Source: CAD feature listing. Evaluate the final solid. Frame: model axes, mm. Face numbers are marked on the shaded views. A direction names the side the tool comes from. Give positions to 0.01 mm unless a question says otherwise; leave off trailing zeros. Write each loop counter-clockwise with the first axis right and the second up, starting at its lowest first coordinate (ties: lowest second). Pieces come first, ordered by that corner, then holes.
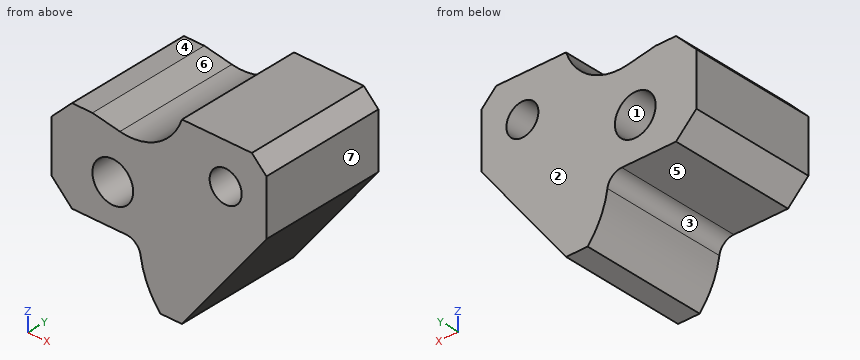
```python
from build123d import *

# Parameters (mm, degrees)
F0_R     = 7
F1_DEPTH = 43
F2_R     = 5.5
F3_DEPTH = 43.001


with BuildPart() as f1:
    # F0 (on Front) → F1 (new body)
    with BuildSketch(Plane.XZ):
        with BuildLine():
            Line((-14, 18), (-21, 11))
            Line((-21, 11), (-21, -7))
            Line((-21, -7), (-14, -14))
            Line((-14, -14), (4.616354, -14))
            ThreePointArc((4.616354, -14), (7.88159, -15.213414), (9.561993, -18.264706))
            ThreePointArc((9.561993, -18.264706), (11.898823, -26.115672), (16.337795, -33))
            Line((16.337795, -33), (23.746698, -33))
            Line((23.746698, -33), (52.746698, 5))
            Line((52.746698, 5), (52.746698, 24))
            Line((52.746698, 24), (47.746698, 29))
            Line((47.746698, 29), (23.746698, 29))
            ThreePointArc((23.746698, 29), (15.440895, 18.713813), (2.43554, 16.33626))
            Line((2.43554, 16.33626), (-7, 18))
            Line((-7, 18), (-14, 18))
        make_face()
        Circle(F0_R, mode=Mode.SUBTRACT)
    extrude(amount=F1_DEPTH)

    # F2 (on face) → F3 (cut, through all)
    with BuildSketch(Plane.XZ.offset(43)):
        with Locations((38.746698, 15)):
            Circle(F2_R)
    extrude(amount=-F3_DEPTH, mode=Mode.SUBTRACT)


solid = f1.part
```
1. Line query: L1, parallel to Z at x = 0, y = -9; L2, parallel to X at y = -34.5, z = 14; L3, parallel to X at y = -15, z = -3. Output: solid intervals per line, ascending.
2. Mould query, pull axis Z, two halves, no side actions, for the marked faces 1, 2 and 3. Classes: +Z half, -Z half, draft (parallel to the pull), parting line (faces both ways), or undercut.
3. Contact query for flat-ended pins moving along their axis: P1, Ø8, axis at y = -33.5, z = -21.5, coming from the -X side; P2, Ø6, axis at x = 44.5, z = 5.5, coming from the +Y side; P3, Ø1.5, axis at x = -4.5, y = -16, coming from the +Z side; P4, Ø10, axis at y = -10, z = -9, coming from the +X side. Output: stop coordinate, or through.
4. Cut plane C-C, the plane x = 0. Return the cut outline in (y, z), then the cut area to 3 significant figures.
5. Cut plane A-A, the plane z = 15. Return the cut outline in (x, y).
6. Cut plane B-B, the plane y = -9.5. Return the cut outline in (x, z), then the cut area to 3 significant figures.
7. Access query for the marked faces 4, 5, 6 and 7. Directions: +Z, -Z, +X, -X, +Y, -Y. A direction counts if a zero-diameter tool reaches every point of the face in a straight line with its end or side. Return the directions, or none.
8. Cut plane D-D, the plane z = -28. Return the cut outline in (x, y), then the cut area to 3 significant figures.
Response values:
1. L1: z = -14 to -7, 7 to 16.77
1. L2: x = -18 to 33.34, 44.16 to 52.75
1. L3: x = -21 to -6.32, 6.32 to 46.64
2. face 1: undercut
2. face 2: draft
2. face 3: -Z half
3. P1: stops at x = 9.39
3. P2: stops at y = 0
3. P3: stops at z = 17.69
3. P4: stops at x = 45.88
4. outline: (-43, -14) - (0, -14) - (0, -7) - (-43, -7) - close; (-43, 7) - (0, 7) - (0, 16.77) - (-43, 16.77) - close
4. area: 721 mm2
5. outline: (-17, -43) - (33.25, -43) - (33.25, 0) - (-17, 0) - close; (44.25, -43) - (52.75, -43) - (52.75, 0) - (44.25, 0) - close
6. outline: (-21, -7) - (-14, -14) - (4.62, -14) arc R5 cw to (9.56, -18.26) arc R29 ccw to (16.34, -33) - (23.75, -33) - (52.75, 5) - (52.75, 24) - (47.75, 29) - (23.75, 29) arc R19 cw to (2.44, 16.34) - (-7, 18) - (-14, 18) - (-21, 11) - close; hole circle Ø14 at (0, 0); hole circle Ø11 at (38.75, 15)
6. area: 2,620 mm2
7. face 4: +Z, -X, +Y, -Y
7. face 5: -Z, -X, +Y, -Y
7. face 6: +Z, +Y, -Y
7. face 7: +Z, -Z, +X, +Y, -Y
8. outline: (12.85, -43) - (27.56, -43) - (27.56, 0) - (12.85, 0) - close
8. area: 633 mm2
